Verification items for this drawing (mm, ordinates from the low corner). A direction names the side the tool comes from. Coordinates: 2 decimals unless noted, no trailing zeros. Order: outer loops, then holes, each group sorted by start corner. A loop starts at its lowest first (then second) coordinate and runs counter-clockwise, first axis right, second up. Notation, with made-up numbers: M 32.25,42 L 48.25,42 A24 cw 48.25,79 Z; hole C 62,12.25 d7. An arc over 180 degrees is marked long. Write item = value, one per line.
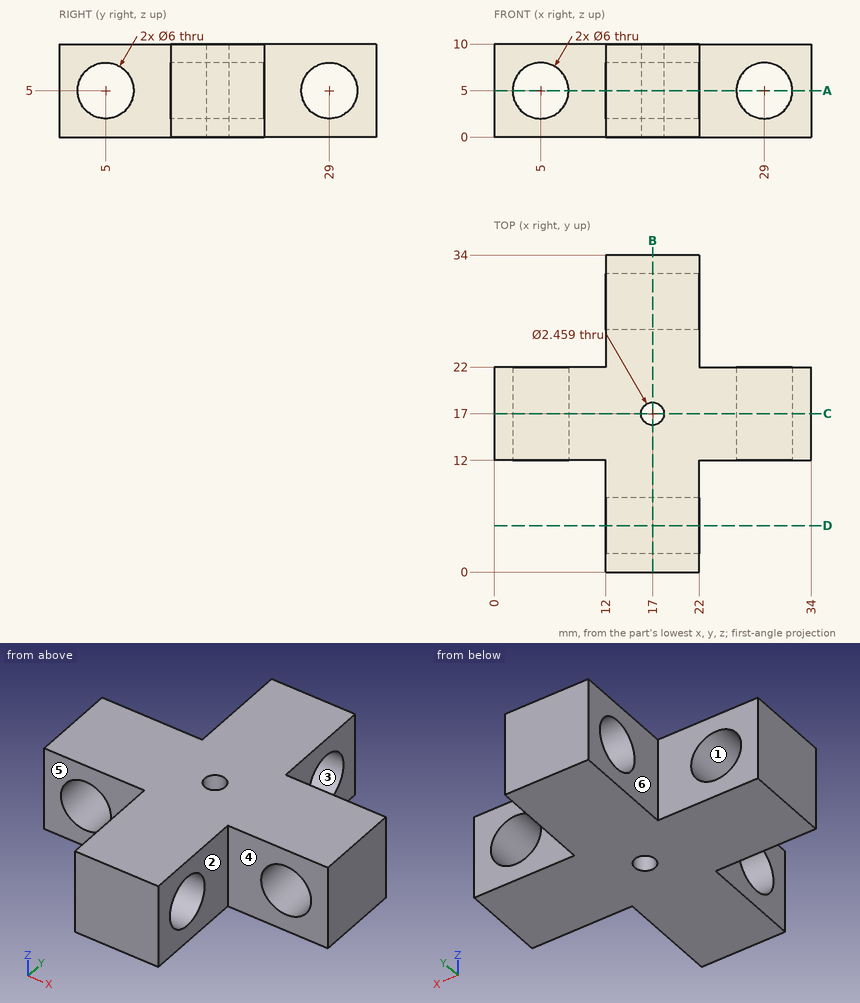
Item 1: Scan lines: L1, parallel to Y at x = 15.25, z = 5; L2, parallel to Y at x = 17, z = 5.5; L3, parallel to X at y = 15, z = 3.75. Record each from-to range of solid material in increasing order. Write a range as from..to.
Report:
L1 = 0..2, 8..26, 32..34
L2 = 0..2.04, 7.96..15.77, 18.23..26.04, 31.96..34
L3 = 0..2.27, 7.73..26.27, 31.73..34
Item 2: Sectioned sample at D-D, the plane y = 5. Enter the section's corners in (x, z).
Report:
outline = M 12,0 L 22,0 L 22,2 L 12,2 Z; M 12,8 L 22,8 L 22,10 L 12,10 Z
Item 3: Release check for a two-part mould opening along X. For the marked faces 1, 2 and 3 record: pulls with the +X half, pulls with the -X half, needs draft (parallel to the pull), parting line crosses it, or undercut.
Report:
face_1 = undercut
face_2 = pulls with the +X half
face_3 = needs draft
Item 4: Sectioned sample at B-B, the plane x = 17. Enter the section's corners in (y, z).
Report:
outline = M 0,0 L 15.77,0 L 15.77,10 L 0,10 Z; M 18.23,0 L 34,0 L 34,10 L 18.23,10 Z; hole C 5,5 d6; hole C 29,5 d6
Item 5: Gauge pin test, flat ends, axial feed: pin 1 (3.5 mm diameter, centred on y = 29, z = 5, fed in from -X); pin 2 (5 mm diameter, centred on x = 29, z = 7, fed in from -Y). Record the tip position at first contact, or that the pin passes through.
Report:
pin_1 = through
pin_2 = 12
Item 6: Sectioned sample at A-A, the plane z = 5. Give the number of separate pieces and of enclosed holes in the cut face, then the cut area to 3 significant figures.
Report:
separate_pieces = 5
enclosed_holes = 1
area = 335 mm^2
Item 7: Tool access check on the marked faces 4, 5 and 6. Record the directions out of +Z, -Z, +X, -X, +Y, -Y that give a thin tool (end or side, any length) a straight path to the whole face; none if there is none.
Report:
face_4 = +Z, -Z, +X, -Y
face_5 = +Z, -Z, -X, -Y
face_6 = +Z, -Z, -X, +Y
